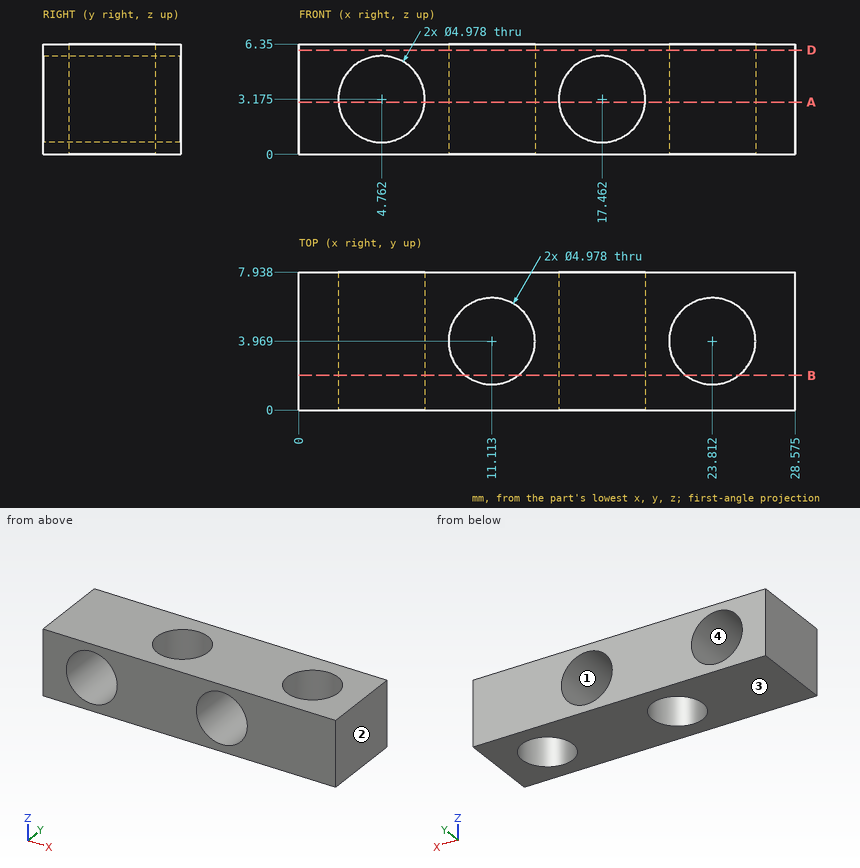
For this review, use the dimensioned drawing (mm, ordinates from the lowest corner) and the shaded views. Give positions to 0.01 mm unless a question says otherwise; leave off trailing zeros. Order: outer loops, then holes, each group sorted by start corner. A loop starts at its lowest first (then second) coordinate and runs counter-clockwise, first axis right, second up. Notation, with made-up numbers: M 76,-8 L 115,-8 A18 ccw 115,24 Z; hole C 68,10 d5. An arc over 180 degrees is marked long. One line per question, with ' | ' between items. Start each with the question number.
1) Wall thickness on L1, parallel to X at y = 7.5, z = 3.75 (1 decimal); L2, parallel to X at y = 7.5, z = 4.75 (1 decimal); L3, parallel to X at y = 3.75, z = 2 (1 decimal): over which ranges is each line inside the solid? List them lowest first. Write a range as from..to.
2) Mouldability with a two-part tool opening along X and no side actions: class the marked faces 1, 2, 3 and 4 as pulls with the +X half, pulls with the -X half, needs draft (parallel to the pull), parting line crosses it, or undercut.
3) Clearance check with a flat-ended pin moving along its axis: P1, Ø3, axis at x = 4.76, z = 3.18, coming from the +Y side. State where the tip first meets the part, or that it passes through.
4) Consider section A-A, the plane z = 3. Give the boundary of the cut face in (x, y) (1 decimal), then the cut area to 3 significant figures.
5) Consider section D-D, the plane z = 6. Give the boundary of the cut face in (x, y) (1 decimal), then the cut area to 3 significant figures.
6) Consider section B-B, the plane y = 2. State how many separate pieces and enclosed holes the cut face has, then the cut area to 3 significant figures.
Found:
1) L1: x = 0..2.3, 7.2..15, 19.9..28.6 | L2: x = 0..2.8, 6.7..15.5, 19.4..28.6 | L3: x = 0..2.6, 7..8.6, 13.6..15.3, 19.7..21.3, 26.3..28.6
2) face 1: undercut | face 2: pulls with the +X half | face 3: needs draft | face 4: undercut
3) P1: passes through
4) outline: M 0,0 L 2.3,0 L 2.3,7.9 L 0,7.9 Z; M 7.2,0 L 15,0 L 15,7.9 L 7.2,7.9 Z; M 19.9,0 L 28.6,0 L 28.6,7.9 L 19.9,7.9 Z; hole C 11.1,4 d5; hole C 23.8,4 d5 | area: 109 mm²
5) outline: M 0,0 L 28.6,0 L 28.6,7.9 L 0,7.9 Z; hole C 11.1,4 d5; hole C 23.8,4 d5 | area: 188 mm²
6) separate pieces: 3 | enclosed holes: 2 | area: 104 mm²
